from build123d import *

# Parameters (mm, degrees)
BOSS_EXTRUDE1_DEPTH = 10
SKETCH29_W          = 20
SKETCH29_H          = 23.5
BOSS_EXTRUDE4_DEPTH = 6.5
SKETCH30_W          = 23.5
SKETCH30_H          = 20
BOSS_EXTRUDE5_DEPTH = 6.5
CHAMFER1_SIZE       = 1
SKETCH4_W           = 21.5
SKETCH4_H           = 5.8
BOSS_EXTRUDE2_DEPTH = 1
SKETCH5_W           = 5.8
SKETCH5_H           = 21.5
BOSS_EXTRUDE3_DEPTH = 1
CHAMFER2_SIZE       = 1


with BuildPart() as part:
    # Sketch2 → Boss-Extrude1 (new, symmetric)
    with BuildSketch(Plane.XY):
        Polygon((-8.159496186, 72.916243655), (70.340503814, -5.583756345), (46.840503814, -5.583756345), (-8.159496186, 49.416243655), align=None)
    extrude(amount=BOSS_EXTRUDE1_DEPTH, both=True)

    # Sketch29 → Boss-Extrude4 (add)
    with BuildSketch(Plane.ZY.offset(8.159496186)):
        with Locations((0, 61.166243655)):
            Rectangle(SKETCH29_W, SKETCH29_H)
    extrude(amount=BOSS_EXTRUDE4_DEPTH)

    # Sketch30 → Boss-Extrude5 (add)
    with BuildSketch(Plane.XZ.offset(5.583756345)):
        with Locations((58.590503814, 0)):
            Rectangle(SKETCH30_W, SKETCH30_H)
    extrude(amount=BOSS_EXTRUDE5_DEPTH)

    # Chamfer1
    chamfer1_edges = [part.edges().sort_by_distance(p)[0] for p in [
        (-11.409496186, 72.916243655, 10),
        (-11.409496186, 72.916243655, -10),
        (-11.409496186, 49.416243655, -10),
        (-11.409496186, 49.416243655, 10),
        (-14.659496186, 72.916243655, 0),
        (-14.659496186, 61.166243655, -10),
        (31.090503814, 33.666243655, 10),
        (-14.659496186, 49.416243655, 0),
        (-14.659496186, 61.166243655, 10),
        (46.840503814, -8.833756345, 10),
        (46.840503814, -8.833756345, -10),
        (70.340503814, -8.833756345, -10),
        (70.340503814, -8.833756345, 10),
        (46.840503814, -12.083756345, 0),
        (58.590503814, -12.083756345, -10),
        (70.340503814, -12.083756345, 0),
        (58.590503814, -12.083756345, 10),
        (31.090503814, 33.666243655, -10),
        (19.340503814, 21.916243655, -10),
        (19.340503814, 21.916243655, 10),
    ]]
    chamfer(chamfer1_edges, length=CHAMFER1_SIZE)

    # Sketch4 → Boss-Extrude2 (add)
    with BuildSketch(Plane.XZ.offset(12.083756345)):
        with Locations((58.590503814, 0)):
            Rectangle(SKETCH4_W, SKETCH4_H)
    extrude(amount=BOSS_EXTRUDE2_DEPTH)

    # Sketch5 → Boss-Extrude3 (add)
    with BuildSketch(Plane.ZY.offset(14.659496186)):
        with Locations((0, 61.166243655)):
            Rectangle(SKETCH5_W, SKETCH5_H)
    extrude(amount=BOSS_EXTRUDE3_DEPTH)

    # Chamfer2
    chamfer2_edges = [part.edges().sort_by_distance(p)[0] for p in [
        (-15.659496186, 61.166243655, 2.9),
        (-15.659496186, 61.166243655, -2.9),
        (58.590503814, -13.083756345, -2.9),
        (58.590503814, -13.083756345, 2.9),
    ]]
    chamfer(chamfer2_edges, length=CHAMFER2_SIZE - 0.0001)  # a hair under: the kernel refuses the full size

    # Sketch34 → CBORE for M3 Hex Socket Head Cap Screw4 (revolve, cut)
    with BuildSketch(Plane(origin=(25.340503814, 61.166243655, 0), x_dir=(0, 0, -1), z_dir=(0, 1, 0))):
        Polygon((0, 0), (0, 41), (1.7, 41), (1.7, 37.425), (1.725, 37.4), (3.25, 37.4), (3.25, 0.025), (3.275, 0), align=None)
    revolve(axis=Axis((31.690503814, 61.166243655, 0), (-1, 0, 0)), mode=Mode.SUBTRACT)

    # Sketch36 → CBORE for M3 Hex Socket Head Cap Screw5 (revolve, cut)
    with BuildSketch(Plane(origin=(58.590503814, 27.916243655, 0), x_dir=(0, 0, 1), z_dir=(1, 0, 0))):
        Polygon((0, 0), (0, 41), (1.7, 41), (1.7, 37.425), (1.725, 37.4), (3.25, 37.4), (3.25, 0.025), (3.275, 0), align=None)
    revolve(axis=Axis((58.590503814, 34.266243655, 0), (0, -1, 0)), mode=Mode.SUBTRACT)


solid = part.part
Input: part model. Units: mm. Frame: model coordinates. A direction names the side the tool comes from. Round coordinates to 2 decimals unless told otherwise and drop trailing zeros. Loops run counter-clockwise (first coordinate to the right, second up) from the corner with the lowest first, then second, coordinate; pieces in that order, holes last. Notation, with made-up numbers: M -26,-38.75 L -21,-38.75 A16 ccw -21,-28.75 Z; hole C -15.75,64 d1. An arc over 180 degrees is marked long. Answer as CSV lines item,"result". Start each with the question number.
(1) Line query: line 1 (Z direction, x = -7, y = 61.5); line 2 (X direction, y = 61.5, z = 5); line 3 (X direction, y = 1.75, z = 0). Output: solid intervals per line, ascending. Write a range as [from, to].
(2) Section A-A, the plane z = -5.25. Output: boundary loops of the cut face in (x, y).
(3) Section B-B, the plane y = 22. Output: boundary loops of the cut face in (x, z).
(4) Section C-C, the plane x = 20. Output: boundary loops of the cut face in (y, z).
(5) Section D-D, the plane z = 0. State how many separate pieces and enclosed holes the cut face has, plus the area to 3 significant figures.
(6) First-contact query: pin 1 (2.5 mm diameter, centred on y = 61.17, z = 0, fed in from -X); pin 2 (4.5 mm diameter, centred on y = -9.5, z = -4, fed in from -X); pin 3 (12 mm diameter, centred on y = 31.5, z = 6, fed in from +X); pin 4 (7 mm diameter, centred on x = 58, z = 0.5, fed in from +Y). Flat tips, straight axial feed; report the tip coordinate or a pass-through.
(7) Reachability of faces 4 (the flat face through (60, -9.484, -1.4)), 5 (the flat face through (58, -12.084, -6)), 6 (the flat face through (58, -12.084, 6)), 7 (the flat face through (-12.059, 63, 1)) from +Z, -Z, +X, -X, +Y, -Y: full face, straight path, thin tool, end or side. Return the list, or none.
(8) Draft query along X for faces 1 (the cylindrical face through (55.368, -2.001, -0.423)), 2 (the flat face through (-11, 49.416, 0)), 3 (the flat face through (-14.659, 61, 6)). Return one class per face: released by +X, released by -X, zero draft, split by the parting line, or undercut.
Values found:
1,line 1,"z = [-10, -3.23], [3.23, 10]"
1,line 2,"x = [-14.66, 3.26]"
1,line 3,"x = [39.51, 55.34], [61.84, 63.01]"
2,outline,"M -14.66,50.42 L -13.66,49.42 L -8.16,49.42 L 46.84,-5.58 L 46.84,-11.08 L 47.84,-12.08 L 69.34,-12.08 L 70.34,-11.08 L 70.34,-5.58 L -8.16,72.92 L -13.66,72.92 L -14.66,71.92 Z"
3,outline,"M 19.26,-9 L 20.67,-10 L 41.34,-10 L 42.76,-9 L 42.76,9 L 41.34,10 L 20.67,10 L 19.26,9 Z"
4,outline,"M 21.26,-9 L 22.67,-10 L 43.34,-10 L 44.76,-9 L 44.76,9 L 43.34,10 L 22.67,10 L 21.26,9 Z"
5,separate pieces,"3"
5,enclosed holes,"0"
5,area,"1,690 mm²"
6,pin 1,"passes through"
6,pin 2,"stops at x = 46.84"
6,pin 3,"stops at x = 39.26"
6,pin 4,"stops at y = 10.26"
7,face 4,"+Y"
7,face 5,"-Z, +X, -X, -Y"
7,face 6,"+Z, +X, -X, -Y"
7,face 7,"+X"
8,face 1,"undercut"
8,face 2,"zero draft"
8,face 3,"released by -X"
